Here's how the part is built. I have some questions about the finished solid (model axes, mm). A direction names the side the tool comes from. Give positions to 0.01 mm unless a question says otherwise; leave off trailing zeros. Loops run counter-clockwise (first coordinate to the right, second up) from the corner with the lowest first, then second, coordinate; pieces in that order, holes last. Notation, with made-up numbers: M 46.25,62 L 70.25,62 A8 cw 70.25,70 Z; hole C 83,-18.5 d11. An arc over 180 degrees is marked long. Write item = value, one per line. Start each with the question number.
```python
from build123d import *

# Parameters (mm, degrees)
ESBO_O1_R                = 4
ESBO_O1_R_2              = 1
ESBO_O1_R_3              = 1.65
RESSALTO_EXTRUS_O1_DEPTH = 3
FILETE1_R                = 20


with BuildPart() as part:
    # Esboço1 → Ressalto-extrusão1 (new body)
    with BuildSketch(Plane.XY):
        with BuildLine():
            Line((14.361406616, -10), (65.638593384, -10))
            ThreePointArc((65.638593384, -10), (97.5, 0), (65.638593384, 10))
            Line((65.638593384, 10), (14.361406616, 10))
            ThreePointArc((14.361406616, 10), (-17.5, 0), (14.361406616, -10))
        make_face()
        Circle(ESBO_O1_R, mode=Mode.SUBTRACT)
        with Locations((-13.25, 0)):
            Circle(ESBO_O1_R_2, mode=Mode.SUBTRACT)
        with Locations((-6.625, 11.4748366)):
            Circle(ESBO_O1_R_2, mode=Mode.SUBTRACT)
        with Locations((86.625, -11.4748366)):
            Circle(ESBO_O1_R_2, mode=Mode.SUBTRACT)
        with Locations((6.625, 11.4748366)):
            Circle(ESBO_O1_R_2, mode=Mode.SUBTRACT)
        with Locations((80, 0)):
            Circle(ESBO_O1_R, mode=Mode.SUBTRACT)
        with Locations((13.25, 0)):
            Circle(ESBO_O1_R_2, mode=Mode.SUBTRACT)
        with Locations((6.625, -11.4748366)):
            Circle(ESBO_O1_R_2, mode=Mode.SUBTRACT)
        with Locations((-6.625, -11.4748366)):
            Circle(ESBO_O1_R_2, mode=Mode.SUBTRACT)
        with Locations((73.375, -11.4748366)):
            Circle(ESBO_O1_R_2, mode=Mode.SUBTRACT)
        with Locations((66.75, 0)):
            Circle(ESBO_O1_R_2, mode=Mode.SUBTRACT)
        with Locations((73.375, 11.4748366)):
            Circle(ESBO_O1_R_2, mode=Mode.SUBTRACT)
        with Locations((86.625, 11.4748366)):
            Circle(ESBO_O1_R_2, mode=Mode.SUBTRACT)
        with Locations((93.25, 0)):
            Circle(ESBO_O1_R_2, mode=Mode.SUBTRACT)
        with Locations((32.5, 0)):
            Circle(ESBO_O1_R_3, mode=Mode.SUBTRACT)
        with Locations((47.5, 0)):
            Circle(ESBO_O1_R_3, mode=Mode.SUBTRACT)
    extrude(amount=RESSALTO_EXTRUS_O1_DEPTH)

    # Filete1
    filete1_edges = [part.edges().sort_by_distance(p)[0] for p in [
        (65.638593384, -10, 1.5),
        (14.361406616, -10, 1.5),
        (14.361406616, 10, 1.5),
        (65.638593384, 10, 1.5),
    ]]
    fillet(filete1_edges, radius=FILETE1_R)


solid = part.part
```
Q1. If I drill on line 1 along Y through (x, z) = (-6.5, 0.65); line 2 along Y through (x, z) = (80, 0.8); line 3 along X through (y, z) = (-2, 1.75), over which ranges is the centre line in solid material (lowest first)?
Q2. We'd pull the mould along Y, two halves only. Please class faces 4 (the flat face through (40, -10, 1)), 5 (the flat face through (40, 10, 1)), 6 (the cylindrical face through (-12.296, 0.3, 1.479)): pulls with the +Y half, pulls with the -Y half, needs draft (parallel to the pull), parting line crosses it, or undercut.
Q3. If we section it at B-B, the plane y = -3: List the corners of the cut face in (x, z) for me, then the cut area to 3 significant figures.
Q4. If we section it at D-D, the plane y = 15: List the corners of the cut face in (x, z) for me, then the cut area to 3 significant figures.
Q5. If we section it at A-A, the plane x = 80: List the corners of the cut face in (y, z) for me, then the cut area to 3 significant figures.
Q6. On a 3-axis mill with a long thin cutter (end or side, diameter ignored), from which of +Z, -Z, +X, -X, +Y, -Y can I reach the whole of each face in a straight line? I mean faces 1 (the cylindrical face through (72.376, 11.519, 1.479)), 2 (the cylindrical face through (63.74, -11, 1.52)), 3 (the cylindrical face through (63.91, 11.055, 1.521)). Say none if no direction works.
Q7. Will these pins go through, and if not, where does the flat tip stop? pin 1 (4.5 mm diameter, centred on x = 32.5, y = 0, fed in from +Z); pin 2 (1.5 mm diameter, centred on x = 31.5, z = 1, fed in from +Y).
Q8. If we section it at C-C, the plane z = 1.4: State how many separate pieces and enclosed holes the cut face has, then the cut area to 3 significant figures.
Resolved:
q1.line_1 = -16.25 to -12.47, -10.48 to 10.48, 12.47 to 16.25
q1.line_2 = -17.5 to -4, 4 to 17.5
q1.line_3 = -17.39 to -3.46, 3.46 to 76.54, 83.46 to 97.39
q2.face_4 = pulls with the -Y half
q2.face_5 = pulls with the +Y half
q2.face_6 = undercut
q3.outline = M -17.24,0 L -2.65,0 L -2.65,3 L -17.24,3 Z; M 2.65,0 L 77.35,0 L 77.35,3 L 2.65,3 Z; M 82.65,0 L 97.24,0 L 97.24,3 L 82.65,3 Z
q3.area = 312 mm²
q4.outline = M -9.01,0 L 9.01,0 L 9.01,3 L -9.01,3 Z; M 70.99,0 L 89.01,0 L 89.01,3 L 70.99,3 Z
q4.area = 108 mm²
q5.outline = M -17.5,0 L -4,0 L -4,3 L -17.5,3 Z; M 4,0 L 17.5,0 L 17.5,3 L 4,3 Z
q5.area = 81.0 mm²
q6.face_1 = +Z, -Z
q6.face_2 = +Z, -Z, -Y
q6.face_3 = +Z, -Z, +Y
q7.pin_1 = 3
q7.pin_2 = 10
q8.separate_pieces = 1
q8.enclosed_holes = 16
q8.area = 2,740 mm²
